Verification items for the finished model (mm, model axes). A direction names the side the tool comes from. Give positions to 0.01 mm unless a question says otherwise; leave off trailing zeros. Write each loop counter-clockwise with the first axis right and the second up, starting at its lowest first coordinate (ties: lowest second). Pieces come first, ordered by that corner, then holes.
from build123d import *

# Parameters (mm, degrees)
SKETCH1_R           = 1.5
SKETCH1_R_2         = 1.65
SKETCH1_W           = 3.48
SKETCH1_H           = 4.16
SKETCH1_R_3         = 2.25
BOSS_EXTRUDE2_DEPTH = 2.1


with BuildPart() as part:
    # Sketch1 → Boss-Extrude2 (new body)
    with BuildSketch(Plane(origin=(0, 0, 0), x_dir=(1, 0, 0), z_dir=(0, 1, 0))):
        Polygon((0, 88.85), (0, 0), (69, 0), (69, -8.5), (82, -8.5), (82, 48), (56, 48), (56, 88.85), (33.24, 88.85), (33.24, 86.17), (29.01, 86.17), (29.01, 88.85), align=None)
        with Locations((3.5, 27.35)):
            Circle(SKETCH1_R, mode=Mode.SUBTRACT)
        with Locations((79, -4.5)):
            Circle(SKETCH1_R_2, mode=Mode.SUBTRACT)
        with Locations((52.5, 27.35)):
            Circle(SKETCH1_R, mode=Mode.SUBTRACT)
        with Locations((3.5, 85.35)):
            Circle(SKETCH1_R, mode=Mode.SUBTRACT)
        with Locations((22.9, 83.58)):
            Rectangle(SKETCH1_W, SKETCH1_H, mode=Mode.SUBTRACT)
        with Locations((37.42, 81.45)):
            Circle(SKETCH1_R_3, mode=Mode.SUBTRACT)
        with Locations((78, 44)):
            Circle(SKETCH1_R_2, mode=Mode.SUBTRACT)
        with BuildLine():
            Line((51.3, 84.45), (51.3, 81.5))
            Line((51.3, 81.5), (47.82, 81.5))
            Line((47.82, 81.5), (47.82, 85.66))
            Line((47.82, 85.66), (51.032382884, 85.66))
            ThreePointArc((51.032382884, 85.66), (52.655843392, 86.841882313), (54, 85.35))
            ThreePointArc((54, 85.35), (52.974341649, 83.926975053), (51.3, 84.45))
        make_face(mode=Mode.SUBTRACT)
    extrude(amount=-BOSS_EXTRUDE2_DEPTH)


solid = part.part
Item 1: Sectioned sample at D-D on z = -44. Record the cut outline in (x, y).
Answer key:
outline: (0, -2.1) - (76.35, -2.1) - (76.35, 0) - (0, 0) - close; (79.65, -2.1) - (82, -2.1) - (82, 0) - (79.65, 0) - close
Item 2: Sectioned sample at C-C on x = 3.5. Record the cut outline in (y, z), then the cut area to 3 significant figures.
Answer key:
outline: (-2.1, -88.85) - (0, -88.85) - (0, -86.85) - (-2.1, -86.85) - close; (-2.1, -83.85) - (0, -83.85) - (0, -28.85) - (-2.1, -28.85) - close; (-2.1, -25.85) - (0, -25.85) - (0, 0) - (-2.1, 0) - close
area: 174 mm2
Item 3: Sectioned sample at B-B on z = -27.35. Record the cut outline in (x, y), then the cut area to 3 significant figures.
Answer key:
outline: (0, -2.1) - (2, -2.1) - (2, 0) - (0, 0) - close; (5, -2.1) - (51, -2.1) - (51, 0) - (5, 0) - close; (54, -2.1) - (82, -2.1) - (82, 0) - (54, 0) - close
area: 160 mm2
Item 4: Scan lines: line 1 along Z through (x, y) = (3.5, -0.9); line 2 along Z through (x, y) = (50, -1.05); line 3 along X through (y, z) = (-0.45, -27.35). Record each from-to range of solid material in increasing order.
Answer key:
line 1: z = -88.85 to -86.85, -83.85 to -28.85, -25.85 to 0
line 2: z = -88.85 to -85.66, -81.5 to 0
line 3: x = 0 to 2, 5 to 51, 54 to 82
Item 5: Sectioned sample at A-A on y = -0.7. State how many separate pieces and enclosed holes the cut face has, then the cut area to 3 significant figures.
Answer key:
separate pieces: 1
enclosed holes: 8
area: 6,230 mm2
Item 6: Release check for a two-part mould opening along Z. For faces 4 (the face through (38.63, -1.035, -83.347)), 5 (the face through (4.19, -1.04, -84.02)), 6 (the face through (29.01, -1, -87)), 7 (the face through (34, -1, 0)) record: released by +Z, released by -Z, zero draft, split by the parting line, or undercut.
Answer key:
face 4: undercut
face 5: undercut
face 6: zero draft
face 7: released by +Z
Item 7: Depth check by flat-ended pin: pin 1 (0.6 mm diameter, centred on y = -1, z = -62.5, fed in from +X); pin 2 (1 mm diameter, centred on y = -2, z = -30.5, fed in from -X); pin 3 (1 mm diameter, centred on y = -1, z = 5, fed in from -X). Enter the tip coordinate at first touch or a pass-through.
Answer key:
pin 1: stops at x = 56
pin 2: stops at x = 0
pin 3: stops at x = 69
Item 8: Set-up check for faces 1 (the face through (31, -1, -86.17)), 2 (the face through (69, -1, -48)), 3 (the face through (21.16, -1, -84)): record each of +Z, -Z, +X, -X, +Y, -Y from which the full face is reachable in a straight line by a thin tool's end or side.
Answer key:
face 1: -Z, +Y, -Y
face 2: -Z, +X, +Y, -Y
face 3: +Y, -Y
